The model under review builds one solid part; all positions refer to its coordinate system, in mm. A direction names the side the tool comes from. Round coordinates to 2 decimals unless told otherwise and drop trailing zeros. Write each loop counter-clockwise with the first axis right and the second up, starting at its lowest first coordinate (ties: lowest second). Pieces come first, ordered by that corner, then holes. Notation, with made-up numbers: (0, 45.25) -> (40, 45.25) arc R15 ccw to (40, 54.25) -> close; hole circle Ø5 at (-21.75, 88). An arc over 180 degrees is marked (long way). Answer as a JSON object with one key per item and string values. Group by question number.
1) We need section B-B, the plane z = 0.45. Write out the cut boundary in (x, y).
2) We need section D-D, the plane x = -10.5. Write out the cut boundary in (y, z), then the cut area to 3 significant figures.
3) Insertion check: pin 1 Ø1.1 at (x, y) = (10, -5.5) entering from +Z; pin 2 Ø0.5 at (y, z) = (0, 0.5) entering from -X. Each pin has a flat end and moves straight along its axis. Give the tip position at first contact, or say it passes through.
4) We need section C-C, the plane y = 7.5. Write out the cut boundary in (x, z).
5) Mouldability with a two-part tool opening along Y and no side actions: class faces 5 (the cylindrical face through (-13.98, 8.61, 0.51)), 6 (the flat face through (-14.731, 6.3, 0.5)), 7 (the cylindrical face through (-14.02, 4.08, 0.51)), 8 (the flat face through (7.3, -4.6, 0.9)) as pulls with the +Y half, pulls with the -Y half, needs draft (parallel to the pull), parting line crosses it, or undercut.
6) We need section A-A, the plane x = 13.5. Write out the cut boundary in (y, z), then the cut area to 3 significant figures.
7) Machinability: for faces 1 (the flat face through (16.269, 2, 0.5)), 2 (the cylindrical face through (-2.3, -4.63, 1.05)), 3 (the flat face through (-8.731, -1, 0.5)), 4 (the flat face through (4, -4, 1.2)), which of the approach directions +Z, -Z, +X, -X, +Y, -Y give a long, thin tool a straight path to every point of the face, cutting with its end or side? Answer none if there is none.
8) To check wall thickness, follow probe 1 along Y at (x, z) = (15.5, 0.9); probe 2 along X at (y, z) = (3, 0.35); probe 3 along X at (y, z) = (-0.25, 0.95). State the ranges of each line that lie inside material, in increasing order. Write a range as [from, to].
from build123d import *

# Parameters (mm, degrees)
SKETCH_W        = 25
SKETCH_H        = 16
PAD_DEPTH       = 1
POCKET_DEPTH    = 0.1
FILLET_R        = 0.75
PAD001_DEPTH    = 0.2
SKETCH003_W     = 5.5
SKETCH003_H     = 2.7
PAD002_DEPTH    = 0.4
SKETCH004_R     = 1.2
POCKET001_DEPTH = 5
SKETCH005_R     = 0.4
POCKET002_DEPTH = 0.2
SKETCH006_R     = 0.4
SKETCH006_R_2   = 0.5
POCKET003_DEPTH = 0.3
SKETCH007_W     = 6
SKETCH007_H     = 1
PAD003_DEPTH    = 6
FILLET001_R     = 2.5
SKETCH008_R     = 1.8
POCKET004_DEPTH = 5


with BuildPart() as part:
    # Sketch → Pad (new body)
    with BuildSketch(Plane.XY):
        with Locations((3.768729, 2.075196)):
            Rectangle(SKETCH_W, SKETCH_H)
    extrude(amount=PAD_DEPTH)

    # Sketch001 (on Face6 of Pad) → Pocket (cut)
    with BuildSketch(Plane.XY.offset(1)):
        with BuildLine():
            Line((-6.731271, 8.975196), (14.268729, 8.975196))
            ThreePointArc((14.768729, 8.475196), (14.622283, 8.82875), (14.268729, 8.975196))
            Line((14.768729, 8.475196), (14.768729, -0.524804))
            ThreePointArc((14.268729, -1.024804), (14.622283, -0.878357), (14.768729, -0.524804))
            Line((14.268729, -1.024804), (-6.731271, -1.024804))
            ThreePointArc((-7.231271, -0.524804), (-7.084824, -0.878357), (-6.731271, -1.024804))
            Line((-7.231271, -0.524804), (-7.231271, 8.475196))
            ThreePointArc((-6.731271, 8.975196), (-7.084824, 8.82875), (-7.231271, 8.475196))
        make_face()
    extrude(amount=-POCKET_DEPTH, mode=Mode.SUBTRACT)

    # Fillet
    fillet_edges = [part.edges().sort_by_distance(p)[0] for p in [
        (-8.731271, 10.075196, 0.5),
        (-8.731271, -5.924804, 0.5),
        (16.268729, -5.924804, 0.5),
        (16.268729, 10.075196, 0.5),
    ]]
    fillet(fillet_edges, radius=FILLET_R)

    # Sketch002 (on Face5 of Fillet) → Pad001 (join)
    with BuildSketch(Plane.XY.offset(1)):
        Polygon((-4.12009, -5.924804), (-3.231271, -2.024804), (10.768729, -2.024804), (11.657549, -5.924804), align=None)
    extrude(amount=PAD001_DEPTH)

    # Sketch003 (on Face24 of Pad001) → Pad002 (join)
    with BuildSketch(Plane.XY.offset(0.9)):
        with BuildLine():
            Line((-3.231271, 5.475196), (10.768729, 5.475196))
            ThreePointArc((11.268729, 4.975196), (11.122283, 5.32875), (10.768729, 5.475196))
            Line((11.268729, 4.975196), (11.268729, 1.475196))
            ThreePointArc((10.768729, 0.975196), (11.122283, 1.121643), (11.268729, 1.475196))
            Line((10.768729, 0.975196), (-3.231271, 0.975196))
            ThreePointArc((-3.731271, 1.475196), (-3.584824, 1.121643), (-3.231271, 0.975196))
            Line((-3.731271, 1.475196), (-3.731271, 4.975196))
            ThreePointArc((-3.231271, 5.475196), (-3.584824, 5.32875), (-3.731271, 4.975196))
        make_face()
        with Locations((3.775376, 3.325196)):
            Rectangle(SKETCH003_W, SKETCH003_H, mode=Mode.SUBTRACT)
    extrude(amount=PAD002_DEPTH)

    # Sketch004 (on Face33 of Pad002) → Pocket001 (cut)
    with BuildSketch(Plane.XY.offset(1.3)):
        with Locations((-1.531271, 3.175196)):
            Circle(SKETCH004_R)
        with Locations((9.068729, 3.175196)):
            Circle(SKETCH004_R)
    extrude(amount=-POCKET001_DEPTH, mode=Mode.SUBTRACT)

    # Sketch005 (on Face5 of Pocket001) → Pocket002 (cut)
    with BuildSketch(Plane.XY.offset(1)):
        with Locations((-7.931271, 9.275196)):
            Circle(SKETCH005_R)
        with Locations((-7.931271, -5.124804)):
            Circle(SKETCH005_R)
        with Locations((15.468729, -5.124804)):
            Circle(SKETCH005_R)
        with Locations((15.468729, 9.275196)):
            Circle(SKETCH005_R)
    extrude(amount=-POCKET002_DEPTH, mode=Mode.SUBTRACT)

    # Sketch006 (on Face30 of Pocket002) → Pocket003 (cut)
    with BuildSketch(Plane.XY.offset(1.2)):
        with Locations((3.768729, -3.424804)):
            Circle(SKETCH006_R)
        with Locations((-2.231271, -5.124804)):
            Circle(SKETCH006_R_2)
        with Locations((9.768729, -5.124804)):
            Circle(SKETCH006_R_2)
        with BuildLine():
            Line((-0.031271, -4.124804), (0.568729, -4.124804))
            ThreePointArc((0.768729, -4.324804), (0.710151, -4.183382), (0.568729, -4.124804))
            Line((0.768729, -4.324804), (0.768729, -4.924804))
            ThreePointArc((0.568729, -5.124804), (0.710151, -5.066225), (0.768729, -4.924804))
            Line((0.568729, -5.124804), (-0.031271, -5.124804))
            ThreePointArc((-0.231271, -4.924804), (-0.172692, -5.066225), (-0.031271, -5.124804))
            Line((-0.231271, -4.924804), (-0.231271, -4.324804))
            ThreePointArc((-0.031271, -4.124804), (-0.172692, -4.183382), (-0.231271, -4.324804))
        make_face()
        with BuildLine():
            Line((7.568729, -4.124804), (6.968729, -4.124804))
            ThreePointArc((6.968729, -4.124804), (6.827308, -4.183382), (6.768729, -4.324804))
            Line((6.768729, -4.324804), (6.768729, -4.924804))
            ThreePointArc((6.768729, -4.924804), (6.827308, -5.066225), (6.968729, -5.124804))
            Line((6.968729, -5.124804), (7.568729, -5.124804))
            ThreePointArc((7.568729, -5.124804), (7.710151, -5.066225), (7.768729, -4.924804))
            Line((7.768729, -4.924804), (7.768729, -4.324804))
            ThreePointArc((7.768729, -4.324804), (7.710151, -4.183382), (7.568729, -4.124804))
        make_face()
    extrude(amount=-POCKET003_DEPTH, mode=Mode.SUBTRACT)

    # Sketch007 (on Face6 of Pocket003) → Pad003 (join)
    with BuildSketch(Plane(origin=(-8.731271, 0, 0), x_dir=(0, -1, 0), z_dir=(-1, 0, 0))):
        with Locations((-6.325196, 0.5)):
            Rectangle(SKETCH007_W, SKETCH007_H)
    extrude(amount=PAD003_DEPTH)

    # Fillet001
    fillet001_edges = [part.edges().sort_by_distance(p)[0] for p in [
        (-14.731271, 3.325196, 0.5),
        (-14.731271, 9.325196, 0.5),
    ]]
    fillet(fillet001_edges, radius=FILLET001_R)

    # Sketch008 (on Face8 of Fillet001) → Pocket004 (cut)
    with BuildSketch(Plane.XY.offset(1)):
        with Locations((-11.731271, 6.325196)):
            Circle(SKETCH008_R)
    extrude(amount=-POCKET004_DEPTH, mode=Mode.SUBTRACT)


solid = part.part
Here are the results:
{
 "1": {"outline": "(-14.73, 5.83) arc R2.5 ccw to (-12.23, 3.33) -> (-8.73, 3.33) -> (-8.73, -5.17) arc R0.75 ccw to (-7.98, -5.92) -> (15.52, -5.92) arc R0.75 ccw to (16.27, -5.17) -> (16.27, 9.33) arc R0.75 ccw to (15.52, 10.08) -> (-7.98, 10.08) arc R0.75 ccw to (-8.73, 9.33) -> (-12.23, 9.33) arc R2.5 ccw to (-14.73, 6.83) -> close; hole circle Ø3.6 at (-11.73, 6.33); hole circle Ø2.4 at (-1.53, 3.18); hole circle Ø2.4 at (9.07, 3.18)"},
 "2": {"outline": "(3.33, 0) -> (5.01, 0) -> (5.01, 1) -> (3.33, 1) -> close; (7.64, 0) -> (9.33, 0) -> (9.33, 1) -> (7.64, 1) -> close", "area": "3.37 mm^2"},
 "3": {"pin 1": "stops at z = 1.2", "pin 2": "stops at x = -8.73"},
 "4": {"outline": "(-14.64, 0) -> (-13.1, 0) -> (-13.1, 1) -> (-14.64, 1) -> close; (-10.37, 0) -> (16.27, 0) -> (16.27, 1) -> (14.77, 1) -> (14.77, 0.9) -> (-7.23, 0.9) -> (-7.23, 1) -> (-10.37, 1) -> close"},
 "5": {"face 5": "pulls with the +Y half", "face 6": "needs draft", "face 7": "pulls with the -Y half", "face 8": "undercut"},
 "6": {"outline": "(-5.92, 0) -> (10.08, 0) -> (10.08, 1) -> (8.98, 1) -> (8.98, 0.9) -> (-1.02, 0.9) -> (-1.02, 1) -> (-5.92, 1) -> close", "area": "15.0 mm^2"},
 "7": {"face 1": "+Z, -Z, +X, +Y, -Y", "face 2": "+Z", "face 3": "+Z, -Z, -X, -Y", "face 4": "+Z, +X, -X, -Y"},
 "8": {"probe 1": "y = [-5.92, -5.52], [-4.73, 8.88], [9.67, 10.08]", "probe 2": "x = [-8.73, -2.72], [-0.34, 7.88], [10.26, 16.27]", "probe 3": "x = [-8.73, -7.23], [14.77, 16.27]"}
}
